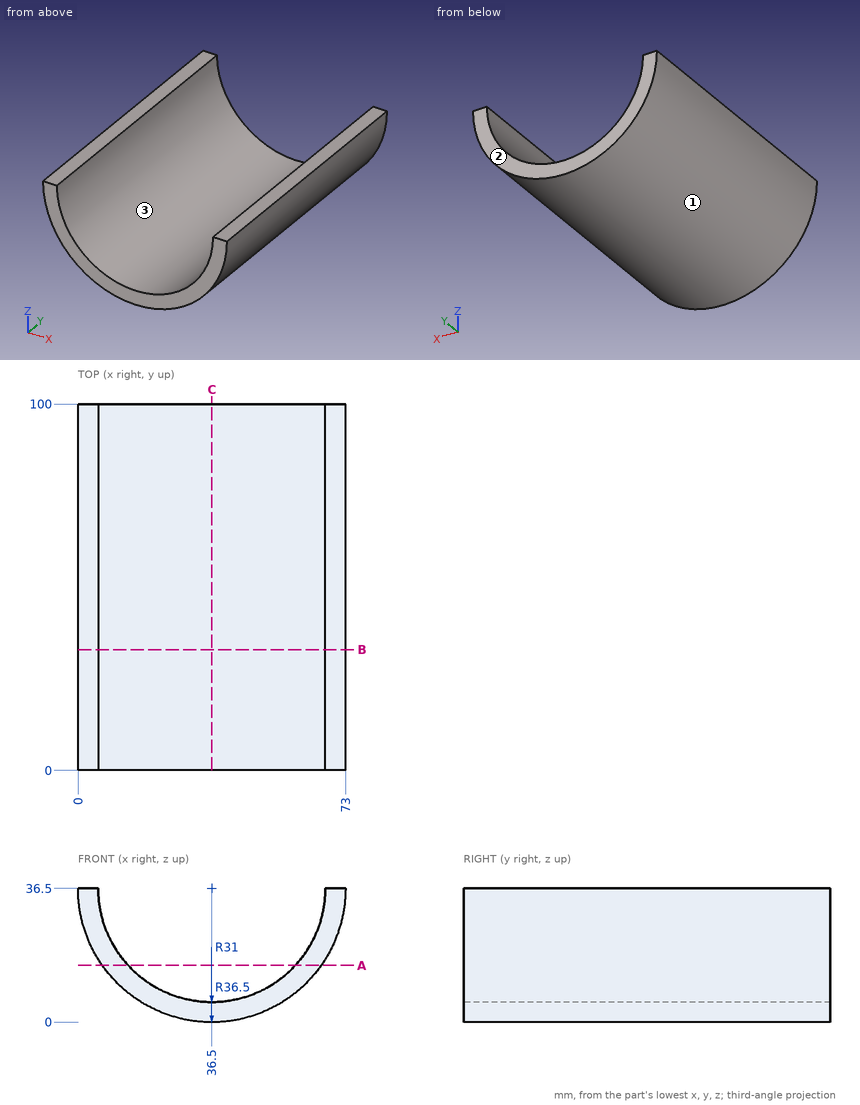
Verification items for this drawing (mm, ordinates from the low corner). Give positions to 0.01 mm unless a question says otherwise; leave off trailing zeros. Write each loop counter-clockwise with the first axis right and the second up, starting at its lowest first coordinate (ties: lowest second). Pieces come first, ordered by that corner, then holes.
1) Gauge pin test, flat ends, axial feed: pin 1 (6 mm diameter, centred on y = 27.5, z = 25.5, fed in from -X); pin 2 (3 mm diameter, centred on x = 19.5, y = 29, fed in from +Z); pin 3 (8 mm diameter, centred on x = 61, y = 58.5, fed in from +Z). Record the tip position at first contact, or that the pin passes through.
2) Material ranges on L1, parallel to X at y = 11, z = 16.5; L2, parallel to X at y = 46, z = 33; L3, parallel to Z at x = 23.5, y = 9.5, recorded low to high.
3) Section check A-A, the plane z = 15.5. Record the boundary of the cut face in (x, y).
4) Section check B-B, the plane y = 33. Record the boundary of the cut face in (x, z), and give its area (3 significant figures).
5) Release check for a two-part mould opening along X. For the marked faces 1, 2 and 3 record: pulls with the +X half, pulls with the -X half, needs draft (parallel to the pull), parting line crosses it, or undercut.
6) Section check C-C, the plane x = 36.5. Record the boundary of the cut face in (y, z), and give its area (3 significant figures).
Computed:
1. pin 1: stops at x = 0.89
1. pin 2: stops at z = 11.63
1. pin 3: stops at z = 24.3
2. L1: x = 5.97 to 12.81, 60.19 to 67.03
2. L2: x = 0.17 to 5.7, 67.3 to 72.83
2. L3: z = 2.39 to 8.36
3. outline: (6.65, 0) - (13.7, 0) - (13.7, 100) - (6.65, 100) - close; (59.3, 0) - (66.35, 0) - (66.35, 100) - (59.3, 100) - close
4. outline: (0, 36.5) arc R36.5 ccw to (73, 36.5) - (67.5, 36.5) arc R31 cw to (5.5, 36.5) - close
4. area: 583 mm2
5. face 1: parting line crosses it
5. face 2: needs draft
5. face 3: undercut
6. outline: (0, 0) - (100, 0) - (100, 5.5) - (0, 5.5) - close
6. area: 550 mm2
